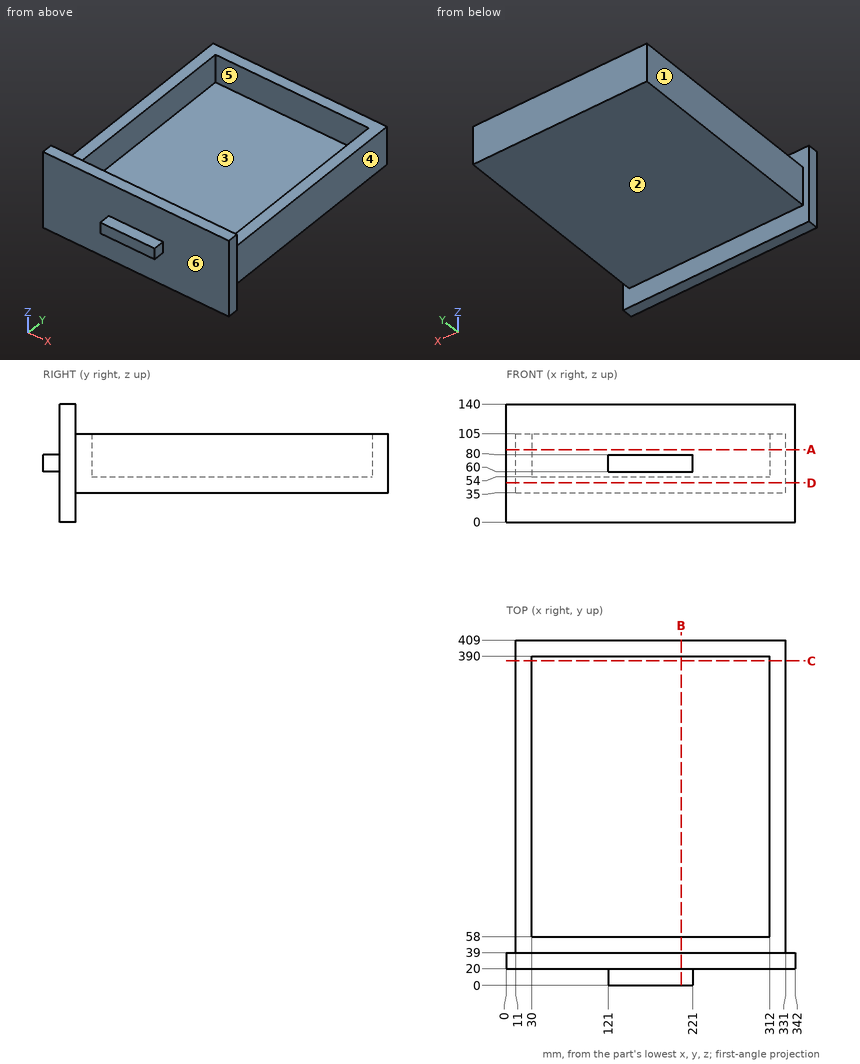
Verification items for this drawing (mm, ordinates from the low corner). A direction names the side the tool comes from. Give positions to 0.01 mm unless a question says otherwise; leave off trailing zeros. Loops run counter-clockwise (first coordinate to the right, second up) from the corner with the lowest first, then second, coordinate; pieces in that order, holes last. Notation, with made-up numbers: M 73.25,-31.75 L 105.25,-31.75 A22 ccw 105.25,3.25 Z; hole C 86,26 d10. An arc over 180 degrees is marked long. Answer as a JSON object with one key per item and string values. Group by question number.
Q1. Access from +Z, -Z, +X, -X, +Y, -Y to the whole of each face (thin tool, end or side, straight path). Record for the marked faces 1, 2 and 3.
Q2. Material ranges on line 1 along Y through (x, z) = (165.5, 85); line 2 along X through (y, z) = (150, 93); line 3 along Y through (x, z) = (170, 19), recorded low to high. Write a range as [from, to].
Q3. Cross-section at D-D on z = 46.5. Record the cut outline in (x, y).
Q4. Release check for a two-part mould opening along X. For the marked faces 4, 5 and 6 record: released by +X, released by -X, zero draft, split by the parting line, or undercut.
Q5. Cross-section at C-C on y = 384.5. Record the cut outline in (x, z).
Q6. Go/stop test with flat-tipped pins: P1, Ø15.5, axis at y = 252, z = 83, coming from the -X side; P2, Ø4, axis at y = 230, z = 85, coming from the +X side; P3, Ø10, axis at x = 193.5, y = 349, coming from the -Z side. Record where each tip stops, or that it passes through.
Q7. Cross-section at A-A on z = 86. Record the cut outline in (x, y).
Q8. Cross-section at B-B on x = 207. Record the cut outline in (y, z), then the cut area to 3 significant figures.
Evaluation:
{
 "1": {"face 1": "+Z, -Z, -X, +Y", "face 2": "-Z, +X, -X, +Y", "face 3": "+Z"},
 "2": {"line 1": "y = [20, 58], [390, 409]", "line 2": "x = [11, 30], [312, 331]", "line 3": "y = [20, 39]"},
 "3": {"outline": "M 0,20 L 342,20 L 342,39 L 331,39 L 331,409 L 11,409 L 11,39 L 0,39 Z"},
 "4": {"face 4": "released by +X", "face 5": "undercut", "face 6": "zero draft"},
 "5": {"outline": "M 11,35 L 331,35 L 331,105 L 312,105 L 312,54 L 30,54 L 30,105 L 11,105 Z"},
 "6": {"P1": "stops at x = 11", "P2": "stops at x = 331", "P3": "stops at z = 35"},
 "7": {"outline": "M 0,20 L 342,20 L 342,39 L 331,39 L 331,409 L 11,409 L 11,39 L 0,39 Z; hole M 30,58 L 312,58 L 312,390 L 30,390 Z"},
 "8": {"outline": "M 0,60 L 20,60 L 20,0 L 39,0 L 39,35 L 409,35 L 409,105 L 390,105 L 390,54 L 58,54 L 58,105 L 39,105 L 39,140 L 20,140 L 20,80 L 0,80 Z", "area": "12,000 mm2"}
}
